Could you check a few things on this model? Use its own coordinates, in mm. Face numbers are marked on the shaded views. A direction names the side the tool comes from. Give positions to 0.01 mm unless a question says otherwise; leave off trailing zeros. Loops run counter-clockwise (first coordinate to the right, second up) from the corner with the lowest first, then second, coordinate; pieces in that order, holes last.
1. Imagine slicing it at A-A (x = 0). List the corners of the cut face in (y, z) for me.
2. I need wall thicknesses on line 1 along Y through (x, z) = (-21, 12); line 2 along Z through (x, y) = (-36, 0.5); line 3 along X through (y, z) = (8.25, 24.5). Which ranges of each line are inside material? Lowest first, please.
3. Imagine slicing it at B-B (z = 9). List the corners of the cut face in (x, y) for me.
4. Imagine slicing it at D-D (z = 16). List the corners of the cut face in (x, y) for me.
5. For the marked faces 1 and 2, which set-ups out of +Z, -Z, +X, -X, +Y, -Y let a thin tool reach every point of the face, with its end or its side?
6. For P1, Ø2.5, axis at x = -42, y = 6.5, coming from the -Z side; P2, Ø10, axis at x = -4.5, z = 7.5, coming from the -Y side; P3, Ø1, axis at y = 3.5, z = -12, coming from the +X side; P4, Ø1, axis at y = -4.5, z = 17, coming from the +X side, each with a flat end and sliding along its axis, tell me the tip position at first contact or that it passes through.
7. Imagine slicing it at C-C (y = -2.25). List the corners of the cut face in (x, z) for me.
```python
from build123d import *

# Parameters (mm, degrees)
SKETCH1_W                = 10
SKETCH1_H                = 30
SKETCH1_W_2              = 70
SKETCH1_H_2              = 60
BOSS_EXTRUDE1_DEPTH      = 10
BOSS_EXTRUDE2_DEPTH      = 10
BOSS_EXTRUDE2_DEPTH_BACK = 20
SKETCH2_W                = 10
SKETCH2_H                = 30
FILLET1_R                = 10
SKETCH3_R                = 5
BOSS_EXTRUDE3_DEPTH      = 5
SKETCH4_W                = 16.278089822
SKETCH4_H                = 6.399401724
CUT_EXTRUDE1_DEPTH       = 5


with BuildPart() as part:
    # Sketch1 → Boss-Extrude1 (new body)
    with BuildSketch(Plane(origin=(0, 0, 0), x_dir=(1, 0, 0), z_dir=(0, 1, 0))):
        with Locations((-40, 0)):
            Rectangle(SKETCH1_W, SKETCH1_H)
        Rectangle(SKETCH1_W_2, SKETCH1_H_2)
    extrude(amount=BOSS_EXTRUDE1_DEPTH)

    # Sketch2 → Boss-Extrude2 (add, two sides: drawn at the far end of the back side and taken through both)
    with BuildSketch(Plane(origin=(0, 10, 0), x_dir=(1, 0, 0), z_dir=(0, 1, 0)).offset(-BOSS_EXTRUDE2_DEPTH_BACK)):
        with Locations((-40, 0)):
            Rectangle(SKETCH2_W, SKETCH2_H)
    extrude(amount=BOSS_EXTRUDE2_DEPTH + BOSS_EXTRUDE2_DEPTH_BACK)

    # Fillet1
    # the kernel refuses this fillet: 10 mm, written as the material it adds along each edge
    with BuildSketch(Plane(origin=(-35, 0, 15), x_dir=(0, -1, 0), z_dir=(0, 0, -1)), Plane(origin=(-35, 10, 15), x_dir=(1, 0, 0), z_dir=(0, 0, -1))) as fillet1_piece_1:
        with BuildLine():
            CenterArc((FILLET1_R, -FILLET1_R), FILLET1_R, 90, 90)
            Line((0, -FILLET1_R), (0, 0))
            Line((0, 0), (FILLET1_R, 0))
        make_face()
    extrude(amount=30)
    # the kernel refuses this fillet: 10 mm, written as the material it takes off along each edge
    with BuildSketch(Plane(origin=(35, 0, -55), x_dir=(0, 1, 0), z_dir=(0, 0, 1))) as fillet1_2_piece_1:
        with BuildLine():
            CenterArc((FILLET1_R, FILLET1_R), FILLET1_R, 180, 90)
            Line((0, FILLET1_R), (0, 0))
            Line((0, 0), (FILLET1_R, 0))
        make_face()
    extrude(amount=110, mode=Mode.SUBTRACT)
    with BuildSketch(Plane(origin=(-35, -25, -30), x_dir=(1, 0, 0), z_dir=(0, 1, 0)), Plane(origin=(35, -25, -30), x_dir=(0, 0, 1), z_dir=(0, 1, 0))) as fillet1_2_piece_2:
        with BuildLine():
            CenterArc((FILLET1_R, -FILLET1_R), FILLET1_R, 90, 90)
            Line((0, -FILLET1_R), (0, 0))
            Line((0, 0), (FILLET1_R, 0))
        make_face()
    extrude(amount=60, mode=Mode.SUBTRACT)
    with BuildSketch(Plane(origin=(35, -25, 30), x_dir=(0, 0, -1), z_dir=(0, 1, 0)), Plane(origin=(-35, -25, 30), x_dir=(1, 0, 0), z_dir=(0, 1, 0))) as fillet1_2_piece_3:
        with BuildLine():
            CenterArc((FILLET1_R, FILLET1_R), FILLET1_R, 180, 90)
            Line((0, FILLET1_R), (0, 0))
            Line((0, 0), (FILLET1_R, 0))
        make_face()
    extrude(amount=60, mode=Mode.SUBTRACT)
    with BuildSketch(Plane(origin=(35, 10, -55), x_dir=(0, -1, 0), z_dir=(0, 0, 1))) as fillet1_2_piece_4:
        with BuildLine():
            CenterArc((FILLET1_R, -FILLET1_R), FILLET1_R, 90, 90)
            Line((0, -FILLET1_R), (0, 0))
            Line((0, 0), (FILLET1_R, 0))
        make_face()
    extrude(amount=110, mode=Mode.SUBTRACT)

    # Sketch3 → Boss-Extrude3 (add)
    with BuildSketch(Plane(origin=(0, 10, 0), x_dir=(1, 0, 0), z_dir=(0, 1, 0))):
        with Locations(Location((0, 15, 0), (0, 0, 270))):
            Circle(SKETCH3_R)
        with Locations(Location((0, -15, 0), (0, 0, 270))):
            Circle(SKETCH3_R)
    extrude(amount=BOSS_EXTRUDE3_DEPTH)

    # Sketch4 → Cut-Extrude1 (cut)
    with BuildSketch(Plane.ZY.offset(45)):
        with Locations((0, 5)):
            Rectangle(SKETCH4_W, SKETCH4_H)
    extrude(amount=-CUT_EXTRUDE1_DEPTH, mode=Mode.SUBTRACT)


solid = part.part
```
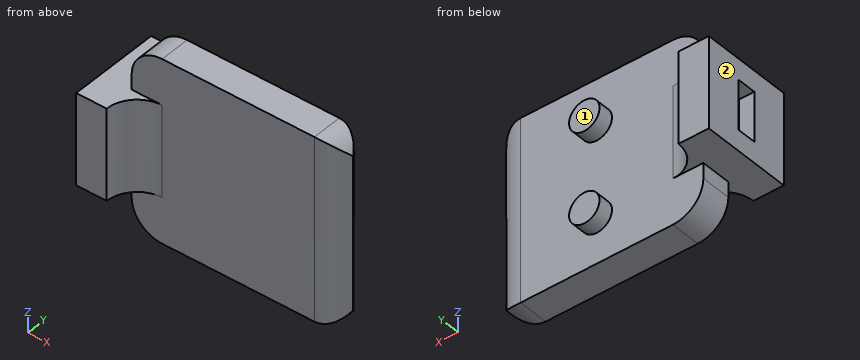
Derived:
1. outline: (0, -30) - (10, -30) - (10, -20) - (15, -20) - (15, -10) - (10, -10) - (10, 10) - (15, 10) - (15, 20) - (10, 20) - (10, 30) - (0, 30) - close
2. line 1: y = 0 to 10
2. line 2: z = -15 to 15
2. line 3: x = -33.93 to 30.65
3. outline: (-45, -10) - (-35, -10) arc R10 cw to (-25, 0) - (25, 0) arc R10 ccw to (33.66, 5) arc R10 ccw to (25, 10) - (-25, 10) arc R10 cw to (-35, 20) - (-45, 20) - close
4. outline: (-35, 0) - (25, 0) arc R10 ccw to (33.66, 5) arc R10 ccw to (25, 10) - (4.9, 10) - (4.9, 15) - (-4.9, 15) - (-4.9, 10) - (-35, 10) - close
5. face 1: +Z, -Z, +X, +Y
5. face 2: +Z, -Z, -X, +Y, -Y
6. P1: stops at z = -15
6. P2: stops at y = 0
6. P3: stops at x = 33
6. P4: passes through
7. outline: (-45, -15) - (-31.32, -15) - (-31.32, 15) - (-45, 15) - close
